```python
from build123d import *

# Parameters (mm, degrees)
BOSS_EXTRUDE1_DEPTH = 92.5
SKETCH2_R           = 1.5
CUT_EXTRUDE1_DEPTH  = 161.2146997
SKETCH4_R           = 1.6
CUT_EXTRUDE2_DEPTH  = 161.214699867
CUT_EXTRUDE3_DEPTH  = 7.5
CUT_EXTRUDE5_DEPTH  = 7.5


with BuildPart() as part:
    # Sketch1 → Boss-Extrude1 (new, symmetric)
    with BuildSketch(Plane.XY):
        with BuildLine():
            ThreePointArc((117.5, 0), (100.658639918, 40.658639918), (60, 57.5))
            Line((60, 57.5), (-60, 57.5))
            ThreePointArc((-60, 57.5), (-100.658639918, 40.658639918), (-117.5, 0))
            Line((-117.5, 0), (-112.5, 0))
            ThreePointArc((-112.5, 0), (-112.485698596, 1.22533379), (-112.442802175, 2.45))
            ThreePointArc((-112.442802175, 2.45), (-112.306489538, 4.503460029), (-112.089802265, 6.55))
            ThreePointArc((-112.089802265, 6.55), (-111.721057974, 9.010114432), (-111.236193262, 11.45))
            ThreePointArc((-111.236193262, 11.45), (-110.731665892, 13.511035335), (-110.144266871, 15.55))
            ThreePointArc((-110.144266871, 15.55), (-91.143819612, 42.264790311), (-60, 52.5))
            Line((-60, 52.5), (-57.05, 52.5))
            Line((-57.05, 52.5), (-52.95, 52.5))
            Line((-52.95, 52.5), (-35.05, 52.5))
            Line((-35.05, 52.5), (-30.95, 52.5))
            Line((-30.95, 52.5), (-13.05, 52.5))
            Line((-13.05, 52.5), (-8.95, 52.5))
            Line((-8.95, 52.5), (8.95, 52.5))
            Line((8.95, 52.5), (13.05, 52.5))
            Line((13.05, 52.5), (30.95, 52.5))
            Line((30.95, 52.5), (35.05, 52.5))
            Line((35.05, 52.5), (52.95, 52.5))
            Line((52.95, 52.5), (57.05, 52.5))
            Line((57.05, 52.5), (60, 52.5))
            ThreePointArc((60, 52.5), (91.143819612, 42.264790311), (110.144266871, 15.55))
            ThreePointArc((110.144266871, 15.55), (110.731665892, 13.511035335), (111.236193262, 11.45))
            ThreePointArc((111.236193262, 11.45), (111.721057974, 9.010114432), (112.089802265, 6.55))
            ThreePointArc((112.089802265, 6.55), (112.306489538, 4.503460029), (112.442802175, 2.45))
            ThreePointArc((112.442802175, 2.45), (112.485698596, 1.22533379), (112.5, 0))
            Line((112.5, 0), (117.5, 0))
        make_face()
    extrude(amount=BOSS_EXTRUDE1_DEPTH, both=True)

    # Sketch2 → Cut-Extrude1 (cut, symmetric)
    with BuildSketch(Plane(origin=(0, 0, 0), x_dir=(0, 0, -1), z_dir=(1, 0, 0))):
        with Locations((-88.75, 4.5)):
            Circle(SKETCH2_R)
        with Locations((-88.75, 13.5)):
            Circle(SKETCH2_R)
    cut_extrude1 = extrude(amount=CUT_EXTRUDE1_DEPTH, both=True, mode=Mode.SUBTRACT)

    # Sketch4 → Cut-Extrude2 (cut, symmetric)
    with BuildSketch(Plane(origin=(0, 57.5, 0), x_dir=(1, 0, 0), z_dir=(0, 1, 0))):
        with Locations(Location((-55, -88.75, 0), (0, 0, 270))):
            Circle(SKETCH4_R)
        with Locations(Location((-33, -88.75, 0), (0, 0, 270))):
            Circle(SKETCH4_R)
        with Locations(Location((-11, -88.75, 0), (0, 0, 270))):
            Circle(SKETCH4_R)
        with Locations(Location((11, -88.75, 0), (0, 0, 270))):
            Circle(SKETCH4_R)
        with Locations(Location((33, -88.75, 0), (0, 0, 270))):
            Circle(SKETCH4_R)
        with Locations(Location((55, -88.75, 0), (0, 0, 270))):
            Circle(SKETCH4_R)
    cut_extrude2 = extrude(amount=CUT_EXTRUDE2_DEPTH, both=True, mode=Mode.SUBTRACT)

    # Sketch5 → Cut-Extrude3 (cut)
    with BuildSketch(Plane(origin=(0, 0, -92.5), x_dir=(-1, 0, 0), z_dir=(0, 0, -1))):
        with BuildLine():
            Line((115.5, 0), (117.5, 0))
            ThreePointArc((117.5, 0), (100.658639918, 40.658639918), (60, 57.5))
            Line((60, 57.5), (-60, 57.5))
            ThreePointArc((-60, 57.5), (-100.658639918, 40.658639918), (-117.5, 0))
            Line((-117.5, 0), (-115.5, 0))
            ThreePointArc((-115.5, 0), (-99.244426356, 39.244426356), (-60, 55.5))
            Line((-60, 55.5), (60, 55.5))
            ThreePointArc((60, 55.5), (99.244426356, 39.244426356), (115.5, 0))
        make_face()
    cut_extrude3 = extrude(amount=-CUT_EXTRUDE3_DEPTH, mode=Mode.SUBTRACT)

    # Mirror1: Cut-Extrude1, Cut-Extrude2, Cut-Extrude3 across plane
    add(cut_extrude1.mirror(Plane.XY), mode=Mode.SUBTRACT)
    add(cut_extrude2.mirror(Plane.XY), mode=Mode.SUBTRACT)
    add(cut_extrude3.mirror(Plane.XY), mode=Mode.SUBTRACT)

    # Sketch6 → Cut-Extrude5 (cut)
    with BuildSketch(Plane(origin=(0, 57.5, 0), x_dir=(1, 0, 0), z_dir=(0, 1, 0))):
        Polygon((-40, 85), (-25, 85), (-25, 92.5), (25, 92.5), (25, 85), (40, 85), (40, -85), (25, -85), (25, -92.5), (-25, -92.5), (-25, -85), (-40, -85), align=None)
    extrude(amount=-CUT_EXTRUDE5_DEPTH, mode=Mode.SUBTRACT)


with BuildPart() as body_2:
    # of the pieces the cut leaves, the one that is kept (cut_extrude5_keep)
    add(part.part.solids().sort_by_distance((-25, 55.5, -92.5))[0])


solid = body_2.part
```
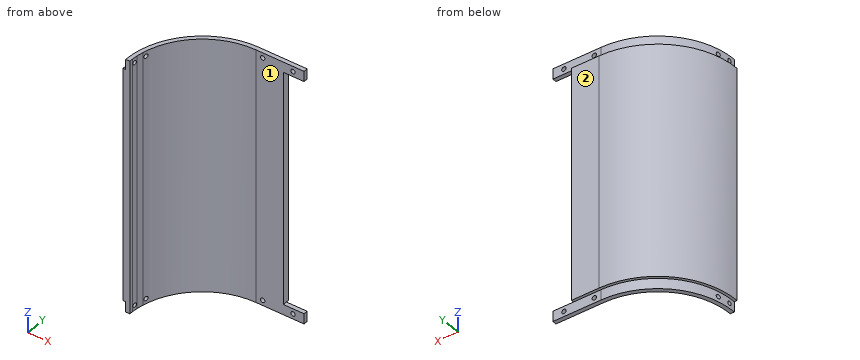
Geometry: final body of the model. Coordinates: model frame, mm. Face numbers are marked on the shaded views. A direction names the side the tool comes from. Give positions to 0.01 mm unless a question says otherwise; leave off trailing zeros. Order: outer loops, then holes, each group sorted by start corner. A loop starts at its lowest first (then second) coordinate and runs counter-clockwise, first axis right, second up. Notation, with made-up numbers: (-18, 28.25) -> (0, 28.25) arc R22 ccw to (0, 52.25) -> close; hole circle Ø3 at (39.25, -9). An arc over 180 degrees is marked (long way). Write each question's results on one line, items separated by ' | '. Start each with the question number.
1) Line query: line 1 (Z direction, x = -111, y = 13); line 2 (Y direction, x = -113.5, z = 88.75); line 3 (Y direction, x = -51, z = 41.5). Output: solid intervals per line, ascending. Write a range as from..to.
2) Section C-C (x = -86). Return loops of the section in (y, z).
3) First-contact query: pin 1 (10 mm diameter, centred on y = 28, z = 22, fed in from -X); pin 2 (6 mm diameter, centred on x = -42.5, z = -89.5, fed in from +Y); pin 3 (6 mm diameter, centred on x = -93, z = -44.5, fed in from +Y); pin 4 (10.5 mm diameter, centred on x = -34, z = -12, fed in from -Y). Flat tips, straight axial feed; report the tip coordinate or a pass-through.
4) Section B-B (x = -107). Return loops of the section in (y, z), then the cut area to 3 significant figures.
5) Set-up query: the marked faces 1 and 2. Return all of +Z, -Z, +X, -X, +Y, -Y with unobstructed straight access to the full face (end or side cutting, diameter ignored); none if empty.
6) Section A-A (z = -28). Return loops of the section in (x, y).
Calculated:
1) line 1: -92.5..-90.16, -87.34..87.34, 90.16..92.5 | line 2: 0..3, 6..12 | line 3: 52.5..57.5
2) outline: (45.61, -92.5) -> (49.03, -92.5) -> (49.03, -85) -> (51.29, -85) -> (51.29, 85) -> (49.03, 85) -> (49.03, 92.5) -> (45.61, 92.5) -> close
3) pin 1: x = -112.7 | pin 2: y = 55.5 | pin 3: y = 49.05 | pin 4: through
4) outline: (23.39, -92.5) -> (29.52, -92.5) -> (29.52, -85) -> (33.12, -85) -> (33.12, 85) -> (29.52, 85) -> (29.52, 92.5) -> (23.39, 92.5) -> close | area: 1,750 mm2
5) face 1: +Z, -Z, +X, -Y | face 2: +Z, -Z, +X, -X, +Y
6) outline: (-117.5, 0) -> (-112.5, 0) arc R52.5 cw to (-60, 52.5) -> (-40, 52.5) -> (-40, 57.5) -> (-60, 57.5) arc R57.5 ccw to start
